Geometry check sheet. Reference: the model listing, model coordinates, mm. Give positions to 0.01 mm unless a question says otherwise; leave off trailing zeros. Loops run counter-clockwise (first coordinate to the right, second up) from the corner with the lowest first, then second, coordinate; pieces in that order, holes last. Notation, with made-up numbers: (79, 15) - (117, 15) arc R22 ccw to (117, 27) - close; hole circle Ø4 at (88, 87.25). An arc over 180 degrees is marked (long way). Use a Markdown table: item, result. Add a question column.
1. Cross-section at D-D on x = 50.5. Enter the section's corners in (y, z).
2. Depth check by flat-ended pin: P1, Ø3, axis at x = 15.5, y = -2.5, coming from the +Z side; P2, Ø1.5, axis at x = 29, y = -7, coming from the -Z side; P3, Ø2, axis at y = -2, z = 198, coming from the +X side. Enter the tip coordinate at first touch or a pass-through.
3. Cross-section at C-C on x = 6.5. Enter the section's corners in (y, z).
4. Material ranges on L1, parallel to X at y = -10.5, z = 88; L2, parallel to X at y = -4.75, z = 161.5; L3, parallel to Z at x = 6.5, y = -2.5, recorded low to high.
5. Cross-section at B-B on y = -8. Enter the section's corners in (x, z).
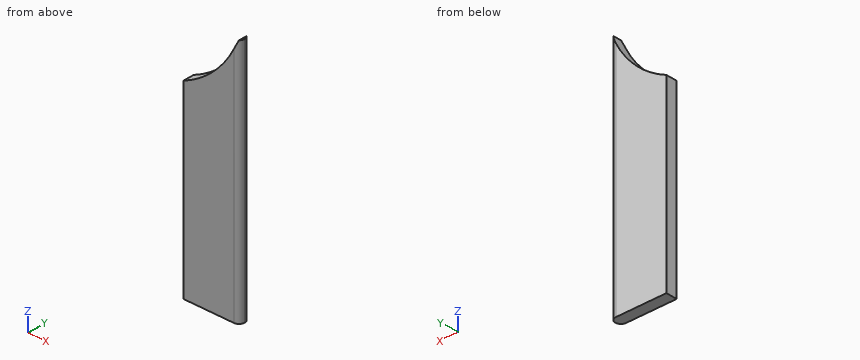
from build123d import *

# Parameters (mm, degrees)
F1_DEPTH = 12
F2_R     = 5.99999


# Not quite as in the source:
# - a fillet or chamfer is up to 0.001 mm smaller than in the source, because OpenCascade refuses the exact size


with BuildPart() as f1:
    # F0 (on Front) → F1 (new body)
    with BuildSketch(Plane.XZ):
        with BuildLine():
            Line((0, 200), (0, 0))
            Line((0, 0), (60, 0))
            Line((60, 0), (60, 260))
            Line((60, 260), (58, 260))
            ThreePointArc((58, 260), (34.9106792543, 224.2863433875), (0, 200))
        make_face()
    extrude(amount=F1_DEPTH)

    # F2 (radius 6 in the source; OpenCascade refuses exactly that, so slightly less here)
    f2_edges = [f1.edges().sort_by_distance(p)[0] for p in [
        (60, -12, 130),
        (60, 0, 130),
    ]]
    fillet(f2_edges, radius=F2_R)


solid = f1.part
Values found:
| question | item | result |
|---|---|---|
| 1 | outline | (-12, 0) - (0, 0) - (0, 244.74) - (-12, 244.74) - close |
| 2 | P1 | stops at z = 209.32 |
| 2 | P2 | stops at z = 0 |
| 2 | P3 | stops at x = 59.2 |
| 3 | outline | (-12, 0) - (0, 0) - (0, 203.11) - (-12, 203.11) - close |
| 4 | L1 | x = 0 to 57.97 |
| 4 | L2 | x = 0 to 59.87 |
| 4 | L3 | z = 0 to 203.11 |
| 5 | outline | (0, 0) - (59.66, 0) - (59.66, 260) - (58, 260) arc R110 cw to (0, 200) - close |
